Read the model definition and answer for the solid it produces. Units are mm, in the model's axes. A direction names the side the tool comes from. Give positions to 0.01 mm unless a question says otherwise; leave off trailing zeros. Loops run counter-clockwise (first coordinate to the right, second up) from the corner with the lowest first, then second, coordinate; pieces in that order, holes last. Notation, with made-up numbers: (-3, 33) -> (3, 33) arc R23 ccw to (3, 44) -> close; hole circle Ø1 at (87, 84.5). An arc over 180 degrees is marked (long way). One line per item, written item: value. Start each with the question number.
from build123d import *

# Parameters (mm, degrees)
CROQUIS1_R              = 1
CROQUIS1_R_2            = 8.5
SALIENTE_EXTRUIR1_DEPTH = 3.5
CROQUIS1_3_R            = 8.5
SALIENTE_EXTRUIR2_DEPTH = 7
REDONDEO1_R             = 1
REDONDEO3_R             = 1


with BuildPart() as part:
    # Croquis1 → Saliente-Extruir1 (new body)
    # profile 1 of 3: a face of its own
    with BuildSketch(Plane(origin=(0, 0, 0), x_dir=(1, 0, 0), z_dir=(0, 1, 0))):
        with BuildLine():
            Line((-2.25, 12.5), (-2.25, 8.196798155))
            ThreePointArc((-2.25, 8.196798155), (0, 8.5), (2.25, 8.196798155))
            Line((2.25, 8.196798155), (2.25, 12.5))
            ThreePointArc((2.25, 12.5), (1.664213562, 13.914213562), (0.25, 14.5))
            Line((0.25, 14.5), (-0.25, 14.5))
            ThreePointArc((-0.25, 14.5), (-1.664213562, 13.914213562), (-2.25, 12.5))
        make_face()
        with Locations(Location((0, 11.5, 0), (0, 0, 270))):
            Circle(CROQUIS1_R, mode=Mode.SUBTRACT)
    # profile 2 of 3: a face of its own
    with BuildSketch(Plane(origin=(0, 0, 0), x_dir=(1, 0, 0), z_dir=(0, 1, 0))):
        Circle(CROQUIS1_R_2)
    # profile 3 of 3: a face of its own
    with BuildSketch(Plane(origin=(0, 0, 0), x_dir=(1, 0, 0), z_dir=(0, 1, 0))):
        with BuildLine():
            ThreePointArc((2.25, -8.196798155), (0, -8.5), (-2.25, -8.196798155))
            Line((-2.25, -8.196798155), (-2.25, -12.5))
            ThreePointArc((-2.25, -12.5), (-1.664213562, -13.914213562), (-0.25, -14.5))
            Line((-0.25, -14.5), (0.25, -14.5))
            ThreePointArc((0.25, -14.5), (1.664213562, -13.914213562), (2.25, -12.5))
            Line((2.25, -12.5), (2.25, -8.196798155))
        make_face()
        with Locations(Location((0, -11.5, 0), (0, 0, 270))):
            Circle(CROQUIS1_R, mode=Mode.SUBTRACT)
    extrude(amount=SALIENTE_EXTRUIR1_DEPTH)

    # Croquis1<3> → Saliente-Extruir2 (add)
    with BuildSketch(Plane(origin=(0, 0, 0), x_dir=(1, 0, 0), z_dir=(0, 1, 0))):
        with Locations(Location((0, 0, 0), (0, 0, 74.650522983))):
            Circle(CROQUIS1_3_R)
    extrude(amount=SALIENTE_EXTRUIR2_DEPTH)

    # Redondeo1
    # the kernel refuses this fillet: 1 mm, written as the material it adds along each edge
    with BuildSketch(Plane(origin=(2.25, 0, -8.196798155), x_dir=(0.9527816834401653, 0, 0.3036561603210522), z_dir=(0, 1, 0)), Plane(origin=(-2.25, 0, 8.196798155), x_dir=(-0.9527816834401646, 0, -0.3036561603210549), z_dir=(0, 1, 0))) as redondeo1_piece_1:
        with BuildLine():
            CenterArc((0.731116518, 0.999174765), REDONDEO1_R, 197.677333553, 69.994809912)
            Line((-0.221665165, 0.695518605), (0, 0))
            ThreePointArc((0, 0), (0.345249467, 0.007014494), (0.690498934, 0))
        make_face()
    extrude(amount=3.5)
    with BuildSketch(Plane(origin=(2.25, 0, 8.196798155), x_dir=(0.9527816834401651, 0, -0.3036561603210529), z_dir=(0, 1, 0)), Plane(origin=(-2.25, 0, -8.196798155), x_dir=(-0.9527816834401648, 0, 0.30365616032105397), z_dir=(0, 1, 0))) as redondeo1_piece_2:
        with BuildLine():
            CenterArc((0.731116518, -0.999174765), REDONDEO1_R, 92.327856536, 69.994809912)
            Line((-0.221665165, -0.695518605), (0, 0))
            ThreePointArc((0, 0), (0.345249467, -0.007014494), (0.690498934, 0))
        make_face()
    extrude(amount=3.5)

    # Croquis2 → Cortar-Revolución1 (revolve, cut)
    with BuildSketch(Plane.XY):
        with BuildLine():
            Line((0, 11.15), (0, 0.85))
            ThreePointArc((0, 0.85), (-5.15, 6), (0, 11.15))
        make_face()
    revolve(axis=Axis((0, 11.15, 0), (0, -1, 0)), mode=Mode.SUBTRACT)

    # Redondeo3
    redondeo3_edges = [part.edges().sort_by_distance(p)[0] for p in [
        (5.05197981, 7, 0),
    ]]
    fillet(redondeo3_edges, radius=REDONDEO3_R)


solid = part.part
Item 1: Section B-B, the plane y = 1.5 is taken. Determine the outline of the cut face in (x, z), plus the area to 3 significant figures.
Item 2: Flat-ended cylindrical pins translate along their axes: pin 1 (1.2 mm diameter, centred on x = 0, z = -11.5, fed in from +Y); pin 2 (1.7 mm diameter, centred on x = -1.5, z = 11, fed in from +Y); pin 3 (4 mm diameter, centred on y = 4, z = 10.5, fed in from +X); pin 4 (1 mm diameter, centred on y = 1.5, z = 11, fed in from +X). Find the tip coordinate at first contact, or state that the pin passes through.
Item 3: Determine the mould class of faces 6 (the cylindrical face through (8.31, 3.45, -1.79)), 7 (the cylindrical face through (-0.6, 1.7, -12.3)), 8 (the flat face through (2.25, 2, -11)) for opening direction Z: pulls with the +Z half, pulls with the -Z half, needs draft (parallel to the pull), parting line crosses it, or undercut.
Item 4: For faces 1 (the flat face through (-2.25, 2, 11)), 2 (the cylindrical face through (2.4, 1.7, -8.4)), 3 (the cylindrical face through (-0.6, 1.7, 10.7)), 4 (the flat face through (2.25, 2, 11)), 5 (the flat face through (-2.25, 2, -11)), determine the directions among +Z, -Z, +X, -X, +Y, -Y from which every point of the face is accessible in a straight line to the end or side of a thin tool.
Item 5: Section D-D, the plane x = 6.75 is taken. Determine the outline of the cut face in (y, z), plus the area to 3 significant figures.
Item 6: Section C-C, the plane y = 4 is taken. Determine the outline of the cut face in (x, z).
Item 7: Consider L1, parallel to X at y = 2.8, z = -11.5; L2, parallel to X at y = 6.5, z = -1.5; L3, parallel to Y at x = -0.75, z = 13. Determine where each line is inside the solid, lowest interval first. Write a range as [from, to].
Item 8: Section A-A, the plane z = 11.5 is taken. Determine the outline of the cut face in (x, y), plus the area to 3 significant figures.
Computed values:
1. outline: (-2.91, -7.99) arc R1 cw to (-2.25, -8.93) -> (-2.25, -12.5) arc R2 ccw to (-0.25, -14.5) -> (0.25, -14.5) arc R2 ccw to (2.25, -12.5) -> (2.25, -8.93) arc R1 cw to (2.91, -7.99) arc R8.5 ccw to (2.91, 7.99) arc R1 cw to (2.25, 8.93) -> (2.25, 12.5) arc R2 ccw to (0.25, 14.5) -> (-0.25, 14.5) arc R2 ccw to (-2.25, 12.5) -> (-2.25, 8.93) arc R1 cw to (-2.91, 7.99) arc R8.5 ccw to start; hole circle Ø5.01 at (0, 0); hole circle Ø2 at (0, -11.5); hole circle Ø2 at (0, 11.5)
1. area: 253 mm²
2. pin 1: through
2. pin 2: y = 3.5
2. pin 3: x = 2.32
2. pin 4: x = 2.25
3. face 6: parting line crosses it
3. face 7: undercut
3. face 8: needs draft
4. face 1: +Z, -X, +Y, -Y
4. face 2: -Z, +X, +Y, -Y
4. face 3: +Y, -Y
4. face 4: +Z, +X, +Y, -Y
4. face 5: -Z, -X, +Y, -Y
5. outline: (0, -5.17) -> (7, -5.17) -> (7, 5.17) -> (0, 5.17) -> close
5. area: 72.3 mm²
6. outline: circle Ø17 at (0, 0); hole circle Ø9.49 at (0, 0)
7. L1: [-2.25, -1], [1, 2.25]
7. L2: [-8.37, -5.07], [5.07, 8.37]
7. L3: [0, 3.5]
8. outline: (-2.25, 0) -> (-1, 0) -> (-1, 3.5) -> (-2.25, 3.5) -> close; (1, 0) -> (2.25, 0) -> (2.25, 3.5) -> (1, 3.5) -> close
8. area: 8.75 mm²
